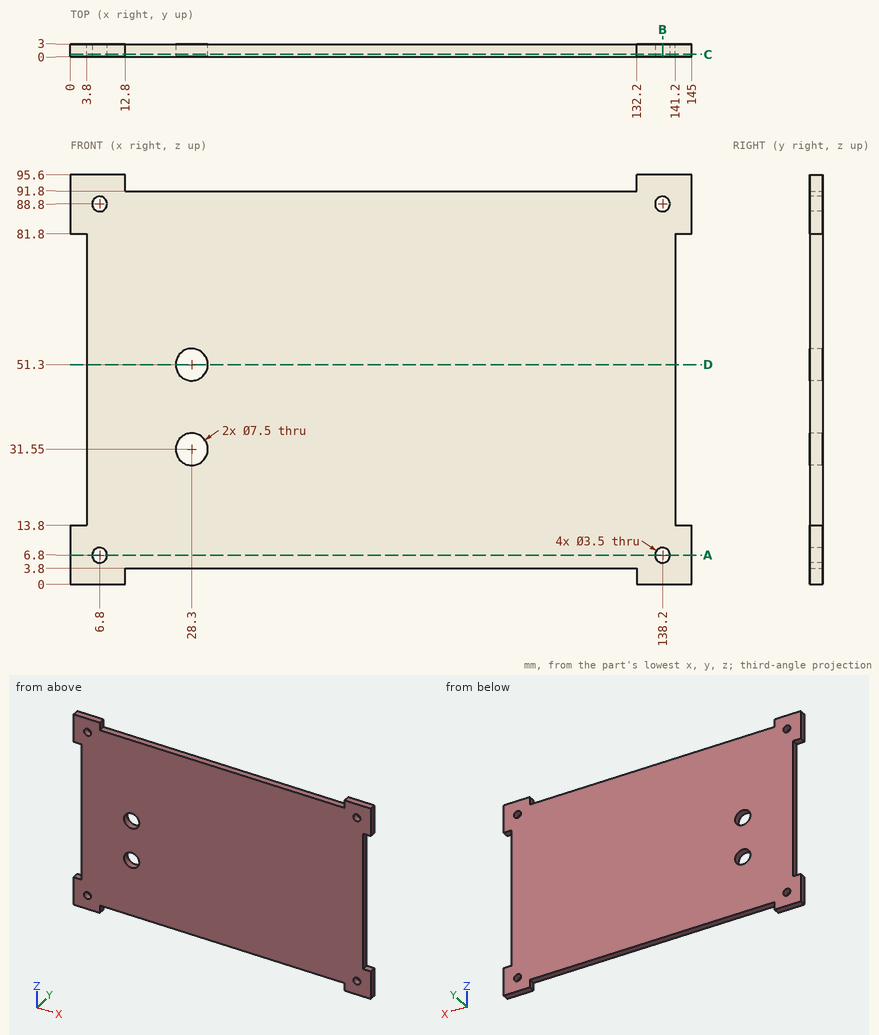
The figure shows three views and two pictorial views of one solid part (mm, origin at its lowest corner). Answer the questions. Coordinates: 2 decimals unless noted, no trailing zeros. Loops run counter-clockwise (first coordinate to the right, second up) from the corner with the lowest first, then second, coordinate; pieces in that order, holes last.
1) Find section B-B on x = 138.2. Write down the section's boundary in (y, z), then the cut area to 3 significant figures.
2) Find section C-C on y = 0.6. Write down the section's boundary in (x, z).
3) Flat-ended cylindrical pins translate along their axes: pin 1 Ø0.9 at (x, y) = (45, 1.5) entering from -Z; pin 2 Ø1.5 at (x, y) = (99, 1.5) entering from +Z; pin 3 Ø1.5 at (y, z) = (2, 54) entering from -X. Find the tip coordinate at first contact, or state that the pin passes through.
4) Find section A-A on z = 6.8. Write down the section's boundary in (x, y), then the cut area to 3 significant figures.
5) Find the intervals of material crossed by L1, parallel to X at y = 0.8, z = 88.8; L2, parallel to Z at x = 6.8, y = 1.9; L3, parallel to Z at x = 93.5, y = 2.45, in increasing order.
6) Find section D-D on z = 51.3. Write down the section's boundary in (x, y).
Values:
1. outline: (0, 0) - (3, 0) - (3, 5.05) - (0, 5.05) - close; (0, 8.55) - (3, 8.55) - (3, 87.05) - (0, 87.05) - close; (0, 90.55) - (3, 90.55) - (3, 95.6) - (0, 95.6) - close
1. area: 266 mm2
2. outline: (0, 0) - (12.8, 0) - (12.8, 3.8) - (132.2, 3.8) - (132.2, 0) - (145, 0) - (145, 13.8) - (141.2, 13.8) - (141.2, 81.8) - (145, 81.8) - (145, 95.6) - (132.2, 95.6) - (132.2, 91.8) - (12.8, 91.8) - (12.8, 95.6) - (0, 95.6) - (0, 81.8) - (3.8, 81.8) - (3.8, 13.8) - (0, 13.8) - close; hole circle Ø3.5 at (6.8, 6.8); hole circle Ø3.5 at (6.8, 88.8); hole circle Ø7.5 at (28.3, 31.55); hole circle Ø7.5 at (28.3, 51.3); hole circle Ø3.5 at (138.2, 6.8); hole circle Ø3.5 at (138.2, 88.8)
3. pin 1: stops at z = 3.8
3. pin 2: stops at z = 91.8
3. pin 3: stops at x = 3.8
4. outline: (0, 0) - (5.05, 0) - (5.05, 3) - (0, 3) - close; (8.55, 0) - (136.45, 0) - (136.45, 3) - (8.55, 3) - close; (139.95, 0) - (145, 0) - (145, 3) - (139.95, 3) - close
4. area: 414 mm2
5. L1: x = 0 to 5.05, 8.55 to 136.45, 139.95 to 145
5. L2: z = 0 to 5.05, 8.55 to 87.05, 90.55 to 95.6
5. L3: z = 3.8 to 91.8
6. outline: (3.8, 0) - (24.55, 0) - (24.55, 3) - (3.8, 3) - close; (32.05, 0) - (141.2, 0) - (141.2, 3) - (32.05, 3) - close
